Autodesk Inventor part; units mm, degrees
ref_plane "YZ Plane" through (0, 0, 0) normal (1, 0, 0) x (0, 1, 0)
ref_plane "XZ Plane" through (0, 0, 0) normal (0, 1, 0) x (-1, 0, 0)
ref_plane "XY Plane" through (0, 0, 0) normal (0, 0, 1) x (1, 0, 0)
sketch "Sketch1" plane through (0, 0, 0) normal (0, 0, 1) x (1, 0, 0)
  line L0 (-95, -10) -> (95, -10)
  line L1 (95, -10) -> (95, 10)
  line L2 (95, 10) -> (-95, 10)
  line L3 (-95, 10) -> (-95, -10)
  line L4 (-95, -10) -> (95, 10) construction
  line L5 (95, -10) -> (-95, 10) construction
  line L6 (-133, 0) -> (133, 0) construction
  line L7 (-83, -5.5) -> (-6, -5.5)
  line L8 (-6, -5.5) -> (-6, 5.5)
  line L9 (-6, 5.5) -> (-83, 5.5)
  line L10 (-83, 5.5) -> (-83, -5.5)
  line L11 (-83, -5.5) -> (-6, 5.5) construction
  line L12 (-6, -5.5) -> (-83, 5.5) construction
  line L13 (0, 14.2899) -> (0, -14.2899) construction
  line L14 (83, -5.5) -> (6, -5.5)
  line L15 (6, -5.5) -> (6, 5.5)
  line L16 (6, 5.5) -> (83, 5.5)
  line L17 (83, 5.5) -> (83, -5.5)
  line L18 (83, -5.5) -> (6, 5.5) construction
  line L19 (6, -5.5) -> (83, 5.5) construction
  circle A0 centre (-89, 0) radius 2.75
  circle A1 centre (0, 0) radius 2.75
  circle A2 centre (89, 0) radius 2.75
  line L20 (6, 5.5) -> (6, 10)
  line L21 (6, -5.5) -> (6, -10)
  point P0 (-44.5, 0)
  point P1 (44.5, 0)
  dimension "d0" = 190
  dimension "d1" = 20
  dimension "d2" = 11
  dimension "d3" = 12
  dimension "d4" = 6
  dimension "d5" = 5.5
  dimension "d6" = 6
  dimension "d7" = 5.5
extrude "Extrusion1" add sketch "Sketch1" along normal blind 4 contours L3 L2 L20 L15 L21 L0
fillet "Fillet1" radius 1 4 edges at (-95, -10, 2) (-95, 10, 2) (6, -10, 2) (6, 10, 2)
sketch "Sketch2" plane through (0, 0, 4) normal (0, 0, 1) x (1, 0, 0)
  arc A0 (6, 9) -> (5, 10) centre (5, 9) ccw
  line L0 (5, 10) -> (-94, 10)
  arc A1 (-94, 10) -> (-95, 9) centre (-94, 9) ccw
  line L1 (-95, 9) -> (-95, -9)
  arc A2 (-95, -9) -> (-94, -10) centre (-94, -9) ccw
  line L2 (-94, -10) -> (5, -10)
  arc A3 (5, -10) -> (6, -9) centre (5, -9) ccw
  line L3 (6, -9) -> (6, 9)
  circle A4 centre (-89, 0) radius 2.75
  circle A5 centre (0, 0) radius 2.75
  line L4 (-83, -5.5) -> (-83, 5.5)
  line L5 (-83, 5.5) -> (-6, 5.5)
  line L6 (-6, 5.5) -> (-6, -5.5)
  line L7 (-6, -5.5) -> (-83, -5.5)
equation "\"d6\" = 0.5 * d3"
equation "\"d7\" = d5"
properties part number "LED_Holder_BackBot"
Here's how the part is built. I have some questions about the finished solid (model axes, mm). A direction names the side the tool comes from. Round coordinates to 2 decimals unless told otherwise and drop trailing zeros. Order: outer loops, then holes, each group sorted by start corner. A loop starts at its lowest first (then second) coordinate and runs counter-clockwise, first axis right, second up. Notation, with made-up numbers: M -2.5,73.25 L 37.5,73.25 A23 cw 37.5,81.25 Z; hole C 11,58.25 d10. An arc over 180 degrees is marked long. Return JSON: item names as keys, results as strings. Group by question number.
1. If we mould it in two halves opening along Y, with no side actions, what happens to faces 3 (the face through (-45, -10, 2)), 4 (the face through (6, 0, 2)), 5 (the face through (-83, 0, 2))? For each: pulls with the +Y half, pulls with the -Y half, needs draft (parallel to the pull), parting line crosses it, or undercut.
2. If we section it at C-C on x = 0: List the corners of the cut face in (y, z) for me, then the cut area to 3 significant figures.
3. On a 3-axis mill with a long thin cutter (end or side, diameter ignored), from which of +Z, -Z, +X, -X, +Y, -Y can I reach the whole of each face in a straight line? I mean faces 1 (the face through (-45, -5.5, 2)), 2 (the face through (-45, 7, 4)). Say none if no direction works.
4. Please list where these lines run through material, in increasing order: probe 1 along Y at (x, z) = (-54.5, 2.6); probe 2 along Y at (x, z) = (0, 1.8); probe 3 along X at (y, z) = (5.25, 1.6).
5. If we section it at B-B on z = 3.3: List the corners of the cut face in (x, y) for me, then the cut area to 3 significant figures.
6. If we section it at A-A on x = -14.5: List the corners of the cut face in (y, z) for me.
7. I'm going to push a flat-ended pin straight in: pin 1 Ø4.5 at (x, y) = (-89, 0) entering from -Z. Where does the tip first touch, or does it pass through?
Reply:
{
 "1": {"face 3": "pulls with the -Y half", "face 4": "needs draft", "face 5": "undercut"},
 "2": {"outline": "M -10,0 L -2.75,0 L -2.75,4 L -10,4 Z; M 2.75,0 L 10,0 L 10,4 L 2.75,4 Z", "area": "58.0 mm^2"},
 "3": {"face 1": "+Z, -Z", "face 2": "+Z, +X, -X, +Y, -Y"},
 "4": {"probe 1": "-10 to -5.5, 5.5 to 10", "probe 2": "-10 to -2.75, 2.75 to 10", "probe 3": "-95 to -83, -6 to 6"},
 "5": {"outline": "M -95,-9 A1 ccw -94,-10 L 5,-10 A1 ccw 6,-9 L 6,9 A1 ccw 5,10 L -94,10 A1 ccw -95,9 Z; hole C -89,0 d5.5; hole M -83,-5.5 L -6,-5.5 L -6,5.5 L -83,5.5 Z; hole C 0,0 d5.5", "area": "1,120 mm^2"},
 "6": {"outline": "M -10,0 L -5.5,0 L -5.5,4 L -10,4 Z; M 5.5,0 L 10,0 L 10,4 L 5.5,4 Z"},
 "7": {"pin 1": "through"}
}
